```python
from build123d import *

# Parameters (mm, degrees)
SKETCH1_R           = 3.2
BOSS_EXTRUDE1_DEPTH = 6.3
FILLET1_R           = 1


with BuildPart() as part:
    # Sketch1 → Boss-Extrude1 (new body)
    with BuildSketch(Plane(origin=(0, 0, 0), x_dir=(1, 0, 0), z_dir=(0, 1, 0))):
        Polygon((-3.681439065, 6.187649506), (-7.199381195, -0.094395), (-3.517942129, -6.282044506), (3.681439065, -6.187649506), (7.199381195, 0.094395), (3.517942129, 6.282044506), align=None)
        with Locations(Location((0, 0, 0), (0, 0, 270))):  # turned: the seam where the file's is
            Circle(SKETCH1_R, mode=Mode.SUBTRACT)
    extrude(amount=BOSS_EXTRUDE1_DEPTH)

    # Fillet1
    fillet1_edges = [part.edges().sort_by_distance(p)[0] for p in [
        (-5.358661662, 6.3, 3.188219753),
        (0.081748468, 6.3, 6.234847006),
        (5.44041013, 6.3, 3.046627253),
        (0, 0, -3.2),
        (0, 6.3, -3.2),
        (5.358661662, 6.3, -3.188219753),
        (-0.081748468, 6.3, -6.234847006),
        (5.358661662, 0, -3.188219753),
        (5.44041013, 0, 3.046627253),
        (0.081748468, 0, 6.234847006),
        (-5.44041013, 6.3, -3.046627253),
        (-5.358661662, 0, 3.188219753),
        (-5.44041013, 0, -3.046627253),
        (-0.081748468, 0, -6.234847006),
    ]]
    fillet(fillet1_edges, radius=FILLET1_R)


solid = part.part
```
Build history of the part. All positions in model axes, mm. A direction names the side the tool comes from. Give positions to 0.01 mm unless a question says otherwise; leave off trailing zeros. Order: outer loops, then holes, each group sorted by start corner. A loop starts at its lowest first (then second) coordinate and runs counter-clockwise, first axis right, second up. Notation, with made-up numbers: M 68,48 L 105,48 A18 cw 105,69 Z; hole C -23.5,21 d3. An arc over 180 degrees is marked long. Return JSON: item names as keys, results as strings.
Q1. Band-saw the part on B-B (y = 6). Give the cut face in (x, z).
Answer list:
{"outline": "M -6.87,0.09 L -3.51,-5.9 L 3.36,-5.99 L 6.87,-0.09 L 3.51,5.9 L -3.36,5.99 Z; hole C 0,0 d6.97"}
Q2. Band-saw the part on A-A (y = 2.25). Give the cut face in (x, z).
Answer list:
{"outline": "M -7.2,0.09 L -3.68,-6.19 L 3.52,-6.28 L 7.2,-0.09 L 3.68,6.19 L -3.52,6.28 Z; hole C 0,0 d6.4"}
Q3. 3-axis set-ups, long thin cutter, end or side, ignore diameter. For faces 1 (the face through (0.13, 6, 5.95)), 2 (the face through (-0.13, 6, -5.95)), 3 (the face through (-0.13, 0.3, -5.95)): which of +Z, -Z, +X, -X, +Y, -Y reach the whole face in a straight line?
Answer list:
{"face 1": "+Z, +X, +Y", "face 2": "-Z, -X, +Y", "face 3": "-Z, -X, -Y"}
Q4. Flat gauge pins, fed straight in: pin 1 (1.5 mm diameter, centred on x = 4.5, y = 2.5, fed in from -Z); pin 2 (1 mm diameter, centred on y = 4.5, z = 2.5, fed in from +X); pin 3 (7.5 mm diameter, centred on x = 0, z = 0, fed in from +Y). Where does each tip first touch, or does it go through?
Answer list:
{"pin 1": "stops at z = -5.89", "pin 2": "stops at x = 6.03", "pin 3": "stops at y = 6.19"}
Q5. Wall check: probe 1 along X at (y, z) = (2.15, 0); probe 2 along X at (y, z) = (5, 0.75); probe 3 along Y at (x, z) = (1.75, -3.75). Give the ranges that are in metal, low to high. Write a range as from..to.
Answer list:
{"probe 1": "x = -7.15..-3.2, 3.2..7.15", "probe 2": "x = -6.81..-3.11, 3.11..6.73", "probe 3": "y = 0..6.3"}
